The listing builds one solid part. Answer for the finished solid, in the listing's coordinates (mm). A direction names the side the tool comes from. Coordinates: 2 decimals unless noted, no trailing zeros. Order: outer loops, then holes, each group sorted by start corner. A loop starts at its lowest first (then second) coordinate and runs counter-clockwise, first axis right, second up. Notation, with made-up numbers: (-27, 21) -> (9, 21) arc R27 cw to (9, 48) -> close; hole circle Ø9 at (-35, 65). An arc over 180 degrees is marked (long way). Return JSON: item names as keys, results as strings.
from build123d import *

# Parameters (mm, degrees)
F0_W     = 1500
F0_H     = 50
F1_DEPTH = 50
F2_W     = 50
F2_H     = 50
F3_DEPTH = 600
F4_W     = 50
F4_H     = 50
F5_DEPTH = 5


with BuildPart() as f1:
    # F0 (on Front) → F1 (new body)
    with BuildSketch(Plane.XZ):
        with Locations((750, -25)):
            Rectangle(F0_W, F0_H)
    extrude(amount=F1_DEPTH)

    # F2 (on face) → F3 (join)
    with BuildSketch(Plane(origin=(0, 0, 0), x_dir=(-1, 0, 0), z_dir=(0, 1, 0))):
        with Locations((-1475, -25)):
            Rectangle(F2_W, F2_H)
    extrude(amount=F3_DEPTH)

    # F4 (on face) → F5 (join)
    with BuildSketch(Plane(origin=(0, 600, 0), x_dir=(-1, 0, 0), z_dir=(0, 1, 0))):
        with BuildLine():
            Line((-1275, 150), (-1475, 150))
            ThreePointArc((-1475, 150), (-1492.67767, 142.67767), (-1500, 125))
            Line((-1500, 125), (-1500, 0))
            Line((-1500, 0), (-1450, 0))
            Line((-1450, 0), (-1450, -50))
            Line((-1450, -50), (-1500, -50))
            Line((-1500, -50), (-1500, -175))
            ThreePointArc((-1500, -175), (-1492.67767, -192.67767), (-1475, -200))
            Line((-1475, -200), (-1275, -200))
            ThreePointArc((-1275, -200), (-1257.32233, -192.67767), (-1250, -175))
            Line((-1250, -175), (-1250, 125))
            ThreePointArc((-1250, 125), (-1257.32233, 142.67767), (-1275, 150))
        make_face()
        with Locations((-1475, -25)):
            Rectangle(F4_W, F4_H)
    extrude(amount=F5_DEPTH)


solid = f1.part
1. Consider line 1 (Y direction, x = 1378.5, z = -38); line 2 (X direction, y = 183, z = -24.5); line 3 (Y direction, x = 1413.5, z = -68.5). Determine where each line is inside the solid, lowest interval first. Write a range as from..to.
Answer block:
{"line 1": "y = -50..0, 600..605", "line 2": "x = 1450..1500", "line 3": "y = 600..605"}
2. The part is cut by section C-C on z = -84. Give the vertices of the cut face in (x, y), and give its area (3 significant figures).
Answer block:
{"outline": "(1250, 600) -> (1500, 600) -> (1500, 605) -> (1250, 605) -> close", "area": "1,250 mm2"}
3. Determine the mould class of faces 1 (the face through (1500, 276, -24)), 2 (the face through (1377, 605, -23)), 3 (the face through (1450, 296, -25)) for opening direction Y: pulls with the +Y half, pulls with the -Y half, needs draft (parallel to the pull), parting line crosses it, or undercut.
Answer block:
{"face 1": "needs draft", "face 2": "pulls with the +Y half", "face 3": "undercut"}
4. Each of these flat-tipped pins is pushed along its axis until it touches: pin 1 Ø8 at (x, z) = (295, -42.5) entering from +Y; pin 2 Ø5.5 at (y, z) = (603, 49.5) entering from -X. Where does it stop, or does it pass through?
Answer block:
{"pin 1": "stops at y = 0", "pin 2": "stops at x = 1250"}
5. The part is cut by section B-B on y = 396. Give the vertices of the cut face in (x, z).
Answer block:
{"outline": "(1450, -50) -> (1500, -50) -> (1500, 0) -> (1450, 0) -> close"}
6. The part is cut by section A-A on x = 1373. Give the vertices of the cut face in (y, z), and give its area (3 significant figures).
Answer block:
{"outline": "(-50, -50) -> (0, -50) -> (0, 0) -> (-50, 0) -> close; (600, -200) -> (605, -200) -> (605, 150) -> (600, 150) -> close", "area": "4,250 mm2"}
7. For faces 4 (the face through (976, -15, 0)), 5 (the face through (976, -15, -50)), 6 (the face through (740, -50, -25)), determine the directions among +Z, -Z, +X, -X, +Y, -Y from which every point of the face is accessible in a straight line to the end or side of a thin tool.
Answer block:
{"face 4": "+Z, +X, -X, -Y", "face 5": "-Z, +X, -X, -Y", "face 6": "+Z, -Z, +X, -X, -Y"}
